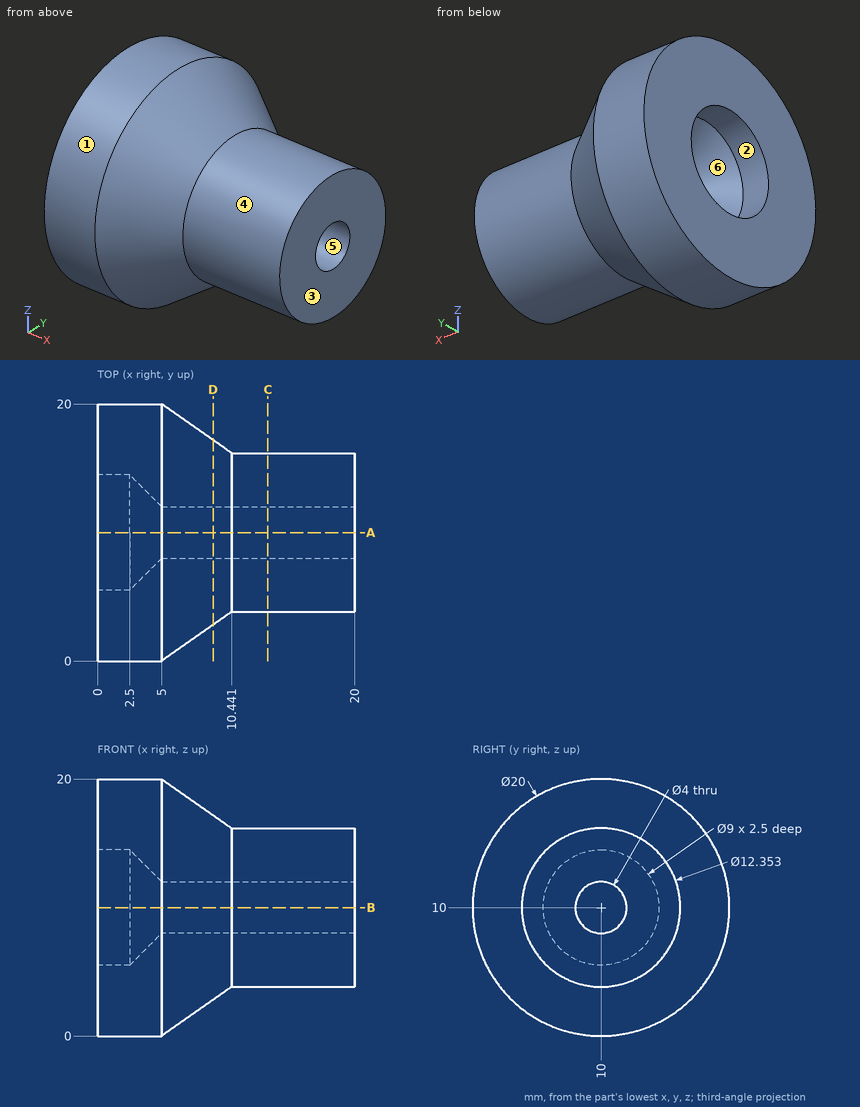
Drawing for the job (mm, zero at the part's lowest x, y, z). A direction names the side the tool comes from. Round coordinates to 2 decimals unless told otherwise and drop trailing zeros. Loops run counter-clockwise (first coordinate to the right, second up) from the corner with the lowest first, then second, coordinate; pieces in that order, holes last. Notation, with made-up numbers: (-1.5, 33) - (23.5, 33) arc R17 cw to (23.5, 45) - close; hole circle Ø3 at (86, 81.25). An arc over 180 degrees is marked (long way). Write each question's results on one line, items separated by ' | '.
(1) Pin check, flat tips, straight feed: pin 1 (5 mm diameter, centred on x = 2.5, z = 5.5, fed in from +Y); pin 2 (6 mm diameter, centred on x = 14, y = 9.5, fed in from +Z); pin 3 (3 mm diameter, centred on x = 4.5, y = 12, fed in from +Z). Stop position of each tip, or through.
Answer below:
pin 1: stops at y = 19.8 | pin 2: stops at z = 16.18 | pin 3: stops at z = 19.99
(2) Saw through at D-D, the plane x = 9. List the corners of the cut face in (y, z).
Answer below:
outline: circle Ø14.38 at (10, 10); hole circle Ø4 at (10, 10)
(3) Saw through at A-A, the plane y = 10. List the corners of the cut face in (x, z), then the cut area to 3 significant figures.
Answer below:
outline: (0, 0) - (5, 0) - (10.44, 3.82) - (20, 3.82) - (20, 8) - (5, 8) - (2.5, 5.5) - (0, 5.5) - close; (0, 14.5) - (2.5, 14.5) - (5, 12) - (20, 12) - (20, 16.18) - (10.44, 16.18) - (5, 20) - (0, 20) - close | area: 207 mm^2
(4) Saw through at C-C, the plane x = 13.25. List the corners of the cut face in (y, z), then the cut area to 3 significant figures.
Answer below:
outline: circle Ø12.35 at (10, 10); hole circle Ø4 at (10, 10) | area: 107 mm^2
(5) Mould opens along Z. For the marked faces 3, 4, 5 and 6 say: released by +Z, released by -Z, zero draft, split by the parting line, or undercut.
Answer below:
face 3: zero draft | face 4: split by the parting line | face 5: undercut | face 6: undercut
(6) 3-axis set-ups, long thin cutter, end or side, ignore diameter. For the marked faces 1 and 2: which of +Z, -Z, +X, -X, +Y, -Y reach the whole face in a straight line?
Answer below:
face 1: +X, -X | face 2: -X
(7) Wall check: L1, parallel to Y at x = 1.35, z = 10; L2, parallel to Z at x = 11.5, y = 11.5; L3, parallel to Z at x = 9, y = 11.5. Give the ranges that are in metal, low to high.
Answer below:
L1: y = 0 to 5.5, 14.5 to 20 | L2: z = 4.01 to 8.68, 11.32 to 15.99 | L3: z = 2.97 to 8.68, 11.32 to 17.03
